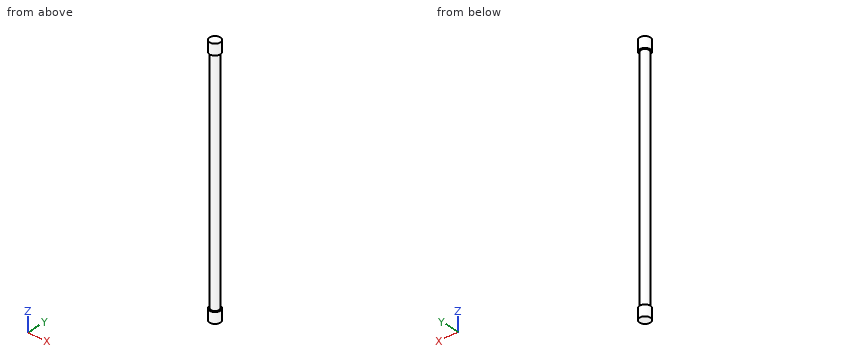
```python
from build123d import *

# Parameters (mm, degrees)
SKETCH1_R           = 7.41
BOSS_EXTRUDE1_DEPTH = 430
SKETCH2_R           = 10
BOSS_EXTRUDE2_DEPTH = 20
SKETCH3_R           = 10
BOSS_EXTRUDE3_DEPTH = 20


with BuildPart() as part:
    # Sketch1 → Boss-Extrude1 (new body)
    with BuildSketch(Plane.XY):
        Circle(SKETCH1_R)
    extrude(amount=-BOSS_EXTRUDE1_DEPTH)

    # Sketch2 → Boss-Extrude2 (add)
    with BuildSketch(Plane(origin=(0, 0, -430), x_dir=(-1, 0, 0), z_dir=(0, 0, -1))):
        Circle(SKETCH2_R)
    extrude(amount=BOSS_EXTRUDE2_DEPTH)

    # Sketch3 → Boss-Extrude3 (add)
    with BuildSketch(Plane.XY):
        Circle(SKETCH3_R)
    extrude(amount=BOSS_EXTRUDE3_DEPTH)


solid = part.part
```
Part model, mm, in its own coordinate system. Round coordinates to 2 decimals unless told otherwise and drop trailing zeros. Loops run counter-clockwise (first coordinate to the right, second up) from the corner with the lowest first, then second, coordinate; pieces in that order, holes last. Notation, with made-up numbers: (70.25, 45.25) -> (121.25, 45.25) arc R19 cw to (121.25, 76.25) -> close; hole circle Ø8 at (77.25, 43.25). An arc over 180 degrees is marked (long way). Use CSV: the item, a comma, the result in double quotes. Start each with the question number.
1) Cut at C-C, the plane z = -390.5. Write the cut outline in (x, y), plus the area to 3 significant figures.
2) Drop flat-ended pins along their axis: P1, Ø5, axis at x = -3, z = -257, coming from the -Y side; P2, Ø5, axis at y = 1, z = -239.5, coming from the -X side; P3, Ø1.5, axis at y = -5, z = -349.5, coming from the +X side. Give the stop position or say it passes through.
3) Cut at A-A, the plane y = 0. Write the cut outline in (x, z), plus the area to 3 significant figures.
4) Wall check: L1, parallel to Z at x = -5, y = 7.75; L2, parallel to Y at x = -0.75, z = -77; L3, parallel to X at y = 0.25, z = -20.5. Give the ranges that are in metal, low to high. Write a range as [from, to].
Determined:
1,outline,"circle Ø14.82 at (0, 0)"
1,area,"172 mm2"
2,P1,"stops at y = -7.39"
2,P2,"stops at x = -7.41"
2,P3,"stops at x = 6.07"
3,outline,"(-10, -450) -> (10, -450) -> (10, -430) -> (7.41, -430) -> (7.41, 0) -> (10, 0) -> (10, 20) -> (-10, 20) -> (-10, 0) -> (-7.41, 0) -> (-7.41, -430) -> (-10, -430) -> close"
3,area,"7,170 mm2"
4,L1,"z = [-450, -430], [0, 20]"
4,L2,"y = [-7.37, 7.37]"
4,L3,"x = [-7.41, 7.41]"
